Autodesk Inventor part; units mm, degrees
ref_plane "YZ Plane" through (0, 0, 0) normal (1, 0, 0) x (0, 1, 0)
ref_plane "XZ Plane" through (0, 0, 0) normal (0, 1, 0) x (-1, 0, 0)
ref_plane "XY Plane" through (0, 0, 0) normal (0, 0, 1) x (1, 0, 0)
sketch "Sketch1" plane through (0, 0, 0) normal (0, 0, 1) x (1, 0, 0)
  circle A0 centre (0, 0) radius 40
  circle A1 centre (0, 0) radius 50
  dimension "d0" = 80
  dimension "d1" = 100
extrude "Extrusion1" add sketch "Sketch1" against normal blind 30
sketch "Sketch2" plane through (0, 0, 0) normal (0, 0, 1) x (1, 0, 0)
  circle A0 centre (0, 0) radius 44.9
  circle A1 centre (0, 0) radius 40
  dimension "d4" = 89.8
extrude "Extrusion2" add sketch "Sketch2" along normal blind 9.25
sketch "Sketch3" plane through (0, 0, 0) normal (0, 1, 0) x (-1, 0, 0)
  point P0 (0, 0)
  point P1 (0, 5)
  dimension "d7" = 5
hole "Hole1" at (0, 0, 5) direction (0, 1, 0) diameter 2.459 end through all
pattern_circular "Circular Pattern1" count 3 over 360 about axis through (0, 0, -10) along (0, 0, 1) of "Hole1"
sketch "Sketch4" plane through (0, 0, 0) normal (0, 1, 0) x (-1, 0, 0)
  point P0 (0, -15)
  point P1 (0, 0)
  dimension "d23" = 15
hole "Hole2" at (0, 0, -15) direction (0, 1, 0) diameter 2.459 end through all counterbore diameter 6.5 counterbore depth 3.4
chamfer "Chamfer1" distance 8 angle 75 1 edges at (-40, 0, -30)
fillet "Fillet1" radius 30 1 edges at (-40, 0, -0.1436)
fillet "Fillet2" radius 1 2 edges at (-48, 0, -30) (-50, 0, -30)
properties part number "Tail"
Here's how the part is built. I have some questions about the finished solid (model axes, mm). A direction names the side the tool comes from. Give positions to 0.01 mm unless a question says otherwise; leave off trailing zeros. Write each loop counter-clockwise with the first axis right and the second up, starting at its lowest first coordinate (ties: lowest second). Pieces come first, ordered by that corner, then holes. Notation, with made-up numbers: (84, 4) -> (135, 4) arc R22 cw to (135, 25) -> close; hole circle Ø2 at (53.25, -22.75). An arc over 180 degrees is marked (long way). Use one line per item in the form item = value. Start each with the question number.
1. On a 3-axis mill with a long thin cutter (end or side, diameter ignored), from which of +Z, -Z, +X, -X, +Y, -Y can I reach the whole of each face in a straight line? I mean faces 4 (the face through (-0.05, 42.48, 6.23)), 5 (the face through (-40.1, -3.1, 9.25)), 6 (the face through (-33.09, -30.35, 4.56)). Say none if no direction works.
2. Thinking about a two-plate mould opening in Z: for faces 1 (the face through (-8.98, 40.46, -5.54)), 2 (the face through (-34, 30, 0)), 3 (the face through (-36.6, -21.56, 3.83)), which applies, +Z half, -Z half, draft (parallel to the pull), parting line (faces both ways), or undercut?
3. If I drill on L1, parallel to X at y = 20.5, z = -20.5; L2, parallel to Y at x = 0, z = 5.6; L3, parallel to Y at x = 12, z = -21, over which ranges is the centre line in solid material (lowest first)?
4. Will these pins go through, and if not, where does the flat tip stop? pin 1 Ø1.5 at (x, z) = (0, 5) entering from -Y; pin 2 Ø8 at (x, z) = (7, -8.5) entering from -Y; pin 3 Ø3 at (y, z) = (-21, 5) entering from -X.
5. Imagine slicing it at C-C on z = -18. List the corners of the cut face in (x, y) for me, plus the area to 3 significant figures.
6. Imagine slicing it at B-B on z = 5. List the corners of the cut face in (x, y) for me.
7. Imagine slicing it at A-A on y = 0. List the corners of the cut face in (x, z) for me.
Entries:
q1.face_4 = +Y
q1.face_5 = +Z, +X, -X, +Y, -Y
q1.face_6 = +Z
q2.face_1 = -Z half
q2.face_2 = +Z half
q2.face_3 = undercut
q3.L1 = -45.6 to -40.57, 40.57 to 45.6
q3.L2 = -44.9 to -40
q3.L3 = -48.54 to -43.98, 43.98 to 48.54
q4.pin_1 = -44.9
q4.pin_2 = -49.91
q4.pin_3 = -40.44
q5.outline = circle Ø100 at (0, 0); hole circle Ø89.57 at (0, 0)
q5.area = 1,550 mm²
q6.outline = (-39.48, -21.38) -> (-35.24, -18.93) arc R40 cw to (-1.23, 39.98) -> (-1.23, 44.88) arc R44.9 ccw to start; (-38.26, -23.51) arc R44.9 ccw to (38.26, -23.51) -> (34.01, -21.06) arc R40 cw to (-34.01, -21.06) -> close; (1.23, 39.98) arc R40 cw to (35.24, -18.93) -> (39.48, -21.38) arc R44.9 ccw to (1.23, 44.88) -> close
q7.outline = (-50, -29) arc R1 ccw to (-49, -30) -> (-48.77, -30) arc R1 ccw to (-47.8, -29.26) -> (-41.02, -3.96) arc R30 ccw to (-40, 3.81) -> (-40, 9.25) -> (-44.9, 9.25) -> (-44.9, 0) -> (-50, 0) -> close; (40, 3.81) arc R30 ccw to (41.02, -3.96) -> (47.8, -29.26) arc R1 ccw to (48.77, -30) -> (49, -30) arc R1 ccw to (50, -29) -> (50, 0) -> (44.9, 0) -> (44.9, 9.25) -> (40, 9.25) -> close
